Design review of the part shown in the three views and the two pictorial views. Dimensions are in mm from the part's minimum x, y and z. Coordinates: 2 decimals unless noted, no trailing zeros. Loops run counter-clockwise (first coordinate to the right, second up) from the corner with the lowest first, then second, coordinate; pieces in that order, holes last. Notation, with made-up numbers: M 50,34 L 55,34 A11 ccw 55,55 Z; hole C 71,19.5 d2. An arc over 180 degrees is marked long. Use one line per item in the form item = value.
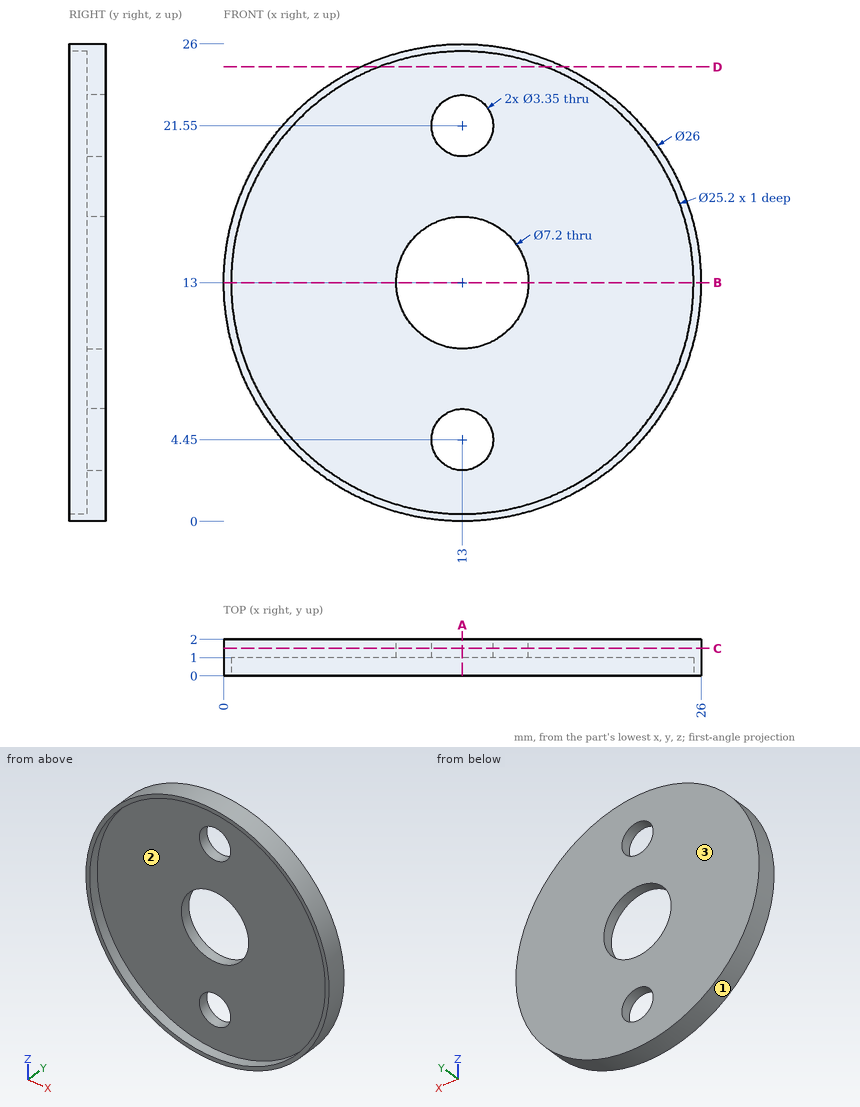
1. Add section B-B (z = 13). State the section outline as (x, y) points.
Response values:
outline = M 0,0 L 0.4,0 L 0.4,1 L 9.4,1 L 9.4,2 L 0,2 Z; M 16.6,1 L 25.6,1 L 25.6,0 L 26,0 L 26,2 L 16.6,2 Z
2. Add section D-D (z = 24.75). State the section outline as (x, y) points, then the cut area to 3 significant figures.
Response values:
outline = M 7.44,0 L 8.45,0 L 8.45,1 L 17.55,1 L 17.55,0 L 18.56,0 L 18.56,2 L 7.44,2 Z
area = 13.1 mm^2
3. Add section C-C (y = 1.5). State the section outline as (x, z) points (3 decimals), then the cut area to 3 significant figures.
Response values:
outline = C 13,13 d26; hole C 13,13 d7.2; hole C 13,4.45 d3.35; hole C 13,21.55 d3.35
area = 473 mm^2
4. Add section A-A (x = 13). State the section outline as (y, z) points (3 decimals), then the cut area to 3 significant figures.
Response values:
outline = M 0,0 L 2,0 L 2,2.775 L 1,2.775 L 1,0.4 L 0,0.4 Z; M 0,25.6 L 1,25.6 L 1,23.225 L 2,23.225 L 2,26 L 0,26 Z; M 1,6.125 L 2,6.125 L 2,9.4 L 1,9.4 Z; M 1,16.6 L 2,16.6 L 2,19.875 L 1,19.875 Z
area = 12.9 mm^2
5. Insertion check: P1, Ø7.5, axis at x = 13.5, z = 8, coming from the -Y side. The pin has a flat end and moves straight along its axis. Give the tip position at first contact, or say it passes through.
Response values:
P1 = 1
6. The part is to be moulded in two halves that separate along Z. For the marked faces 1, 2 and 3, say which applies: pulls with the +Z half, pulls with the -Z half, needs draft (parallel to the pull), parting line crosses it, or undercut.
Response values:
face_1 = parting line crosses it
face_2 = undercut
face_3 = needs draft
7. Wall thickness on line 1 along Z through (x, y) = (12.5, 1.3); line 2 along Y through (x, z) = (1.5, 12.25); line 3 along X through (y, z) = (1.5, 13): over which ranges is each line inside the solid? List them lowest first. Write a range as from..to.
Response values:
line_1 = 0.01..2.85, 6.05..9.43, 16.57..19.95, 23.15..25.99
line_2 = 1..2
line_3 = 0..9.4, 16.6..26
